Read the model definition and answer for the solid it produces. Units are mm, in the model's axes. A direction names the side the tool comes from. Coordinates: 2 decimals unless noted, no trailing zeros. Loops run counter-clockwise (first coordinate to the right, second up) from the corner with the lowest first, then second, coordinate; pieces in that order, holes last. Notation, with made-up numbers: M -13.5,40.5 L -4.5,40.5 A30 ccw -4.5,79.5 Z; hole C -5.75,-13 d5. An arc over 180 degrees is marked long. One line per item, written item: value. Start each with the question number.
1. A flat-ended cylindrical pin translates along its axis: pin 1 (2 mm diameter, centred on x = 6.5, y = 3.5, fed in from +Z). Find the tip coordinate at first contact, or state that the pin passes through.
2. For faces 1 (the face through (10, 5, 0)), 2 (the face through (10, 5, 13)), determine the directions among +Z, -Z, +X, -X, +Y, -Y from which every point of the face is accessible in a straight line to the end or side of a thin tool.
3. Consider probe 1 along Z at (x, y) = (5.25, 6.25); probe 2 along X at (y, z) = (2.5, 11.5). Determine where each line is inside the solid, lowest interval first.
4. The part is cut by section B-B (x = 8.75). Write down the section's boundary in (y, z), then the cut area to 3 significant figures.
5. The part is cut by section C-C (z = 12.5). Write down the section's boundary in (x, y).
6. The part is cut by section A-A (y = 4). Write down the section's boundary in (x, z), then the cut area to 3 significant figures.
```python
from build123d import *

# Parameters (mm, degrees)
BOX001_W     = 10
BOX001_H     = 10
BOX001_DEPTH = 16
BOX_W        = 10
BOX_H        = 10
BOX_DEPTH    = 10


with BuildPart() as cube001:
    # Box001 → Box001 (new body)
    with BuildSketch(Plane(origin=(10, 0, 0), x_dir=(1, 0, 0), z_dir=(0, 0, 1))):
        with Locations((5, 5)):
            Rectangle(BOX001_W, BOX001_H)
    extrude(amount=BOX001_DEPTH)


with BuildPart() as fusion:
    # Box → Box (new body)
    with BuildSketch(Plane.XY):
        with Locations((5, 5)):
            Rectangle(BOX_W, BOX_H)
    extrude(amount=BOX_DEPTH)

    # Fusion: union Cube001
    add(cube001.part)


solid = fusion.part
```
Answer block:
1. pin 1: stops at z = 10
2. face 1: -Z, +X, -X, +Y, -Y
2. face 2: +Z, -X, +Y, -Y
3. probe 1: z = 0 to 10
3. probe 2: x = 10 to 20
4. outline: M 0,0 L 10,0 L 10,10 L 0,10 Z
4. area: 100 mm2
5. outline: M 10,0 L 20,0 L 20,10 L 10,10 Z
6. outline: M 0,0 L 20,0 L 20,16 L 10,16 L 10,10 L 0,10 Z
6. area: 260 mm2
